Autodesk Inventor part; units mm, degrees
ref_plane "YZ Plane" through (0, 0, 0) normal (1, 0, 0) x (0, 1, 0)
ref_plane "XZ Plane" through (0, 0, 0) normal (0, 1, 0) x (-1, 0, 0)
ref_plane "XY Plane" through (0, 0, 0) normal (0, 0, 1) x (1, 0, 0)
sketch "Sketch1" plane through (0, 0, 0) normal (0, 0, 1) x (1, 0, 0)
  line L0 (-44.45, 127) -> (44.45, 127)
  line L1 (44.45, 127) -> (44.45, 50.8)
  line L2 (-44.45, 50.8) -> (-44.45, 127)
  line L3 (31.75, 50.8) -> (31.75, 0)
  line L4 (31.75, 0) -> (-31.75, 0)
  line L5 (-31.75, 0) -> (-31.75, 50.8)
  line L6 (-44.45, 50.8) -> (-31.75, 50.8)
  line L7 (31.75, 50.8) -> (44.45, 50.8)
  line L8 (152.4, 0) -> (-152.4, 0) construction
  point P0 (0, 0)
  dimension "d0" = 88.9
  dimension "d1" = 76.2
  dimension "d3" = 44.45
  dimension "d4" = 63.5
  dimension "d12" = 152.4
  dimension "d13" = 152.4
revolve "Snow Blower Tire" add sketch "Sketch1" angle 360 about axis through (31.75, 0, 0) along (-1, 0, 0)
fillet "Fillet1" radius 25.4 2 edges at (44.45, -127, 0) (-44.45, -127, 0)
chamfer "Chamfer1" distance 12.7 angle 45 2 edges at (44.45, -50.8, 0) (-44.45, -50.8, 0)
sketch "Sketch21" plane through (0, 0, 0) normal (0, 1, 0) x (-1, 0, 0)
  line L0 (83.9649, 0) -> (-81.8871, 0)
  point P0 (0, 0)
properties part number "Snow Blower Tire"
Design review of the part built by this model. Coordinates are the model's own, in mm. A direction names the side the tool comes from. Give positions to 0.01 mm unless a question says otherwise; leave off trailing zeros. Write each loop counter-clockwise with the first axis right and the second up, starting at its lowest first coordinate (ties: lowest second). Pieces come first, ordered by that corner, then holes. Notation, with made-up numbers: (-36, -26) - (-8, -26) arc R21 cw to (-8, -16) - close; hole circle Ø3 at (26, 89.25). An arc over 180 degrees is marked (long way). Return JSON: item names as keys, results as strings. Group by question number.
(1) Insertion check: pin 1 (5 mm diameter, centred on x = -20, y = 22.5, fed in from +Z); pin 2 (1.5 mm diameter, centred on x = 23, z = -8.5, fed in from -Y); pin 3 (4 mm diameter, centred on x = -27, y = 47.5, fed in from -Z). Each pin has a flat end and moves straight along its axis. Give the tip position at first contact, or say it passes through.
(2) We need section D-D, the plane x = 36. Give the boundary of the cut face in (y, z).
(3) We need section C-C, the plane x = -7.5. Give the boundary of the cut face in (y, z).
(4) To check wall thickness, follow probe 1 along Z at (x, y) = (-31.8, 0); probe 2 along X at (y, z) = (26.5, -7.5). State the ranges of each line that lie inside material, in increasing order.
(5) Machinability: for faces 1 (the flat face through (-44.45, -47, 44)), 2 (the flat face through (-31.75, -1, -1)), which of the approach directions +Z, -Z, +X, -X, +Y, -Y give a long, thin tool a straight path to every point of the face, cutting with its end or side? Answer none if there is none.
(6) Mouldability with a two-part tool opening along Y and no side actions: class faces 3 (the flat face through (44.45, -47, 44)), 4 (the flat face through (31.75, -1, -1)), 5 (the cylindrical face through (0.27, -27.53, -123.98)), 6 (the conical face through (32.545, 49.212, 15.498)) as +Y half, -Y half, draft (parallel to the pull), parting line (faces both ways), or undercut.
Reported:
{
 "1": {"pin 1": "stops at z = 125.4", "pin 2": "stops at y = -126.52", "pin 3": "stops at z = -117.44"},
 "2": {"outline": "circle Ø241.03 at (0, 0); hole circle Ø110.1 at (0, 0)"},
 "3": {"outline": "circle Ø254 at (0, 0)"},
 "4": {"probe 1": "z = -123.57 to -50.85, 50.85 to 123.57", "probe 2": "x = -31.75 to 31.75"},
 "5": {"face 1": "+Z, -Z, -X, +Y, -Y", "face 2": "-X"},
 "6": {"face 3": "draft", "face 4": "undercut", "face 5": "parting line", "face 6": "undercut"}
}
